from build123d import *

# Parameters (mm, degrees)
BOSS_EXTRUDE1_DEPTH = 60
SKETCH6_W           = 76.2
SKETCH6_H           = 139.7
BOSS_EXTRUDE3_DEPTH = 3
SKETCH7_W           = 254.695348458
SKETCH7_H           = 135.329086622
CUT_EXTRUDE1_DEPTH  = 76.2
SKETCH8_W           = 10
SKETCH8_H           = 5
CUT_EXTRUDE2_DEPTH  = 172.74190537
SKETCH9_W           = 55
SKETCH9_H           = 40
CUT_EXTRUDE3_DEPTH  = 246.885251985
SKETCH10_W          = 200.764393162
SKETCH10_H          = 14.388440844
CUT_EXTRUDE4_DEPTH  = 15
BOSS_EXTRUDE4_DEPTH = 4
BOSS_EXTRUDE5_DEPTH = 4
SKETCH13_W          = 162.798604232
SKETCH13_H          = 246.735608635
CUT_EXTRUDE5_DEPTH  = 101.6


with BuildPart() as part:
    # Sketch1 → Boss-Extrude1 (new body)
    with BuildSketch(Plane.XY):
        with BuildLine():
            Line((-101.6, 101.6), (-101.6, -38.1))
            ThreePointArc((-101.6, -38.1), (-83.001280605, -83.001280605), (-38.1, -101.6))
            Line((-38.1, -101.6), (38.1, -101.6))
            ThreePointArc((38.1, -101.6), (83.001280605, -83.001280605), (101.6, -38.1))
            Line((101.6, -38.1), (101.6, 101.6))
            Line((101.6, 101.6), (-101.6, 101.6))
        make_face()
        with BuildLine():
            Line((-98.6, 98.6), (-98.6, -38.1))
            ThreePointArc((-98.6, -38.1), (-80.879960262, -80.879960262), (-38.1, -98.6))
            Line((-38.1, -98.6), (38.1, -98.6))
            ThreePointArc((38.1, -98.6), (80.879960262, -80.879960262), (98.6, -38.1))
            Line((98.6, -38.1), (98.6, 98.6))
            Line((98.6, 98.6), (-98.6, 98.6))
        make_face(mode=Mode.SUBTRACT)
    extrude(amount=BOSS_EXTRUDE1_DEPTH)

    # Sweep2: sweep along a path in Sketch5
    with BuildLine(Plane.XY.offset(60)) as sweep2_path:
        Line((-100.1, 101.6), (-100.1, -38.1))
        ThreePointArc((-100.1, -38.1), (-81.940620434, -81.940620434), (-38.1, -100.1))
        Line((-38.1, -100.1), (38.1, -100.1))
        ThreePointArc((38.1, -100.1), (81.940620434, -81.940620434), (100.1, -38.1))
        Line((100.1, -38.1), (100.1, 101.6))
    # Sketch3 → Sweep2 (sweep)
    with BuildSketch(Plane(origin=(0, 101.6, 0), x_dir=(1, 0, 0), z_dir=(0, 1, 0))):
        with BuildLine():
            Line((-38.1, -91.039099262), (-88.9, -91.039099262))
            ThreePointArc((-88.9, -91.039099262), (-95.981959893, -87.480761361), (-98.6, -80))
            Line((-98.6, -80), (-98.6, -60))
            Line((-98.6, -60), (-101.6, -60))
            Line((-101.6, -60), (-101.6, -80))
            ThreePointArc((-101.6, -80), (-98.157592659, -89.649805752), (-88.9, -94.039099262))
            Line((-88.9, -94.039099262), (-38.1, -94.039099262))
            Line((-38.1, -94.039099262), (-38.1, -91.039099262))
        make_face()
    sweep(path=sweep2_path.line)

    # Sketch6 → Boss-Extrude3 (add)
    with BuildSketch(Plane.XY.offset(94.039099262)):
        with Locations((0, 31.75)):
            Rectangle(SKETCH6_W, SKETCH6_H)
    extrude(amount=-BOSS_EXTRUDE3_DEPTH)

    # Sketch7 → Cut-Extrude1 (cut)
    with BuildSketch(Plane(origin=(0, 101.6, 0), x_dir=(1, 0, 0), z_dir=(0, 1, 0))):
        with Locations((-4.889183354, -23.374555951)):
            Rectangle(SKETCH7_W, SKETCH7_H)
    extrude(amount=-CUT_EXTRUDE1_DEPTH, mode=Mode.SUBTRACT)

    # Sketch8 → Cut-Extrude2 (cut, through all)
    with BuildSketch(Plane.XY.offset(94.039099262)):
        with Locations((0, 39.440517612)):
            Rectangle(SKETCH8_W, SKETCH8_H)
    extrude(amount=-CUT_EXTRUDE2_DEPTH, mode=Mode.SUBTRACT)

    # Sketch9 → Cut-Extrude3 (cut, through all)
    with BuildSketch(Plane(origin=(0, -101.6, 0), x_dir=(-1, 0, 0), z_dir=(0, -1, 0))):
        with Locations((0, -20)):
            Rectangle(SKETCH9_W, SKETCH9_H)
    extrude(amount=-CUT_EXTRUDE3_DEPTH, mode=Mode.SUBTRACT)

    # Sketch10 → Cut-Extrude4 (cut)
    with BuildSketch(Plane(origin=(0, 101.6, 0), x_dir=(1, 0, 0), z_dir=(0, 1, 0))):
        with Locations((0, -94.039099262)):
            Rectangle(SKETCH10_W, SKETCH10_H)
    extrude(amount=-CUT_EXTRUDE4_DEPTH, mode=Mode.SUBTRACT)

    # Sketch11 → Boss-Extrude4 (add)
    with BuildSketch(Plane(origin=(0, -98.6, 0), x_dir=(1, 0, 0), z_dir=(0, 1, 0))):
        Polygon((0, -80), (1.5, -80), (1.5, -40), (0, -40), (-1.5, -40), (-1.5, -80), align=None)
    extrude(amount=BOSS_EXTRUDE4_DEPTH)

    # Sketch12 → Boss-Extrude5 (add)
    with BuildSketch(Plane(origin=(0, 0, 91.039099262), x_dir=(-1, 0, 0), z_dir=(0, 0, -1))):
        Polygon((-1.5, -88.9), (0, -88.9), (1.5, -88.9), (1.5, 36.940517612), (-1.5, 36.940517612), align=None)
    extrude(amount=BOSS_EXTRUDE5_DEPTH)

    # Sketch13 → Cut-Extrude5 (cut)
    with BuildSketch(Plane.ZY.offset(101.6)):
        with Locations((24.668934791, -31.353857456)):
            Rectangle(SKETCH13_W, SKETCH13_H)
    extrude(amount=-CUT_EXTRUDE5_DEPTH, mode=Mode.SUBTRACT)


with BuildPart() as cut_extrude5_kept_piece:
    # of the separate pieces the step leaves, the one the design keeps (cut_extrude5_pieces_kept)
    add(part.part.solids().sort_by_distance((0, 86.6, 91.039099262))[0])


solid = cut_extrude5_kept_piece.part
Read the model definition and answer for the solid it produces. Units are mm, in the model's axes. A direction names the side the tool comes from. Round coordinates to 2 decimals unless told otherwise and drop trailing zeros. Order: outer loops, then holes, each group sorted by start corner. A loop starts at its lowest first (then second) coordinate and runs counter-clockwise, first axis right, second up.
1) The part is cut by section A-A on x = 25. Write down the section's boundary in (y, z), plus the area to 3 significant figures.
2) Straight lines are drawn through the part: L1, parallel to X at y = -15, z = 19; L2, parallel to Y at x = 20, z = 50; L3, parallel to Z at x = 28, y = 62.5. For each, find the intervals that lie inside material, in ascending order.
3) The part is cut by section C-C on y = 15.5. Write down the section's boundary in (x, z).
4) Flat-ended cylindrical pins translate along their axes: pin 1 (1.5 mm diameter, centred on y = 23, z = 44.5, fed in from -X); pin 2 (1.5 mm diameter, centred on y = -99.5, z = 21, fed in from -X); pin 3 (1.6 mm diameter, centred on x = 1, y = -96.5, fed in from +Z). Find the tip coordinate at first contact, or state that the pin passes through.
5) The part is cut by section B-B on z = 43.5. Write down the section's boundary in (x, y), plus the area to 3 significant figures.
6) The mould has two halves that part along X. Classify faces 1 (the face through (48, 0, 91.039)), 2 (the face through (19.317, -98.058, 89.758)), 3 (the face through (0, -42, 89)): released by +X, released by -X, zero draft, split by the parting line, or undercut.
7) The part is cut by section D-D on z = 16. Write down the section's boundary in (x, y), plus the area to 3 significant figures.
8) For faces 4 (the face through (1.5, -25, 89)), 5 (the face through (98.6, -6, 41)), 6 (the face through (14, -100, 40)), 7 (the face through (1.9, 36.941, 91.4)), determine the directions among +Z, -Z, +X, -X, +Y, -Y from which every point of the face is accessible in a straight line to the end or side of a thin tool.
Resolved:
1. outline: (-101.6, 40) - (-98.6, 40) - (-98.6, 80) arc R10.57 cw to (-88.9, 91.04) - (86.6, 91.04) - (86.6, 94.04) - (-88.9, 94.04) arc R13.39 ccw to (-101.6, 80) - close
1. area: 703 mm2
2. L1: x = 98.6 to 101.6
2. L2: y = -101.6 to -98.6
2. L3: z = 91.04 to 94.04
3. outline: (0, 87.04) - (1.5, 87.04) - (1.5, 91.04) - (88.9, 91.04) arc R10.57 cw to (98.6, 80) - (98.6, 0) - (101.6, 0) - (101.6, 80) arc R13.39 ccw to (88.9, 94.04) - (0, 94.04) - close
4. pin 1: stops at x = 98.6
4. pin 2: stops at x = 27.5
4. pin 3: stops at z = 91.78
5. outline: (0, -101.6) - (38.1, -101.6) arc R63.5 ccw to (101.6, -38.1) - (101.6, 25.4) - (98.6, 25.4) - (98.6, -38.1) arc R60.5 cw to (38.1, -98.6) - (1.5, -98.6) - (1.5, -94.6) - (0, -94.6) - close
5. area: 603 mm2
6. face 1: undercut
6. face 2: zero draft
6. face 3: released by -X
7. outline: (27.5, -101.6) - (38.1, -101.6) arc R63.5 ccw to (101.6, -38.1) - (101.6, 25.4) - (98.6, 25.4) - (98.6, -38.1) arc R60.5 cw to (38.1, -98.6) - (27.5, -98.6) - close
7. area: 514 mm2
8. face 4: -Z, +Y
8. face 5: -Z, -X, +Y
8. face 6: -Z, -X, +Y, -Y
8. face 7: +Z, -Z, -X
